Part model, mm, in its own coordinate system. Face numbers are marked on the shaded views. A direction names the side the tool comes from. Round coordinates to 2 decimals unless told otherwise and drop trailing zeros. Loops run counter-clockwise (first coordinate to the right, second up) from the corner with the lowest first, then second, coordinate; pieces in that order, holes last. Notation, with made-up numbers: M 61.25,7 L 81.25,7 A22 ccw 81.25,22 Z; hole C -36,14.25 d2. An arc over 180 degrees is marked long. Answer as CSV lines item,"result". Start each with the question number.
Item 1: Which spindle directions (+Z, -Z, +X, -X, +Y, -Y) get a long thin tool onto all of the face, cutting with end or side? Do the marked faces 4 and 5. Say none if no direction does.
Item 2: Band-saw the part on D-D (z = 5.25). Give the cut face in (x, y).
Item 3: Band-saw the part on C-C (z = 0.5). Give the cut face in (x, y), and give its area (3 significant figures).
Item 4: Band-saw the part on A-A (x = 0). Give the cut face in (y, z), and give its area (3 significant figures).
Item 5: Wall check: line 1 (Y direction, x = 0, z = 2); line 2 (Z direction, x = -4.75, y = -4.25); line 3 (Z direction, x = -4.75, y = 5). Give the ranges that are in metal, low to high.
Item 6: Mould opens along Y. For the marked faces 1, 2 and 3 say: pulls with the +Y half, pulls with the -Y half, needs draft (parallel to the pull), parting line crosses it, or undercut.
Item 7: Drop flat-ended pins along their axis: pin 1 Ø2 at (x, z) = (-4, 1.5) entering from +Y; pin 2 Ø1 at (y, z) = (-4.5, -1.5) entering from -X; pin 3 Ø2 at (x, z) = (2, -3) entering from +Y. Give the stop position or say it passes through.
```python
from build123d import *


with BuildPart() as f1:
    # F0 (on Front) → F1 (revolve)
    with BuildSketch(Plane.XZ):
        Polygon((-1.8, -6), (-1.8, 0), (-4.8, 0), (-4.8, -2.8), (-4.8, -6), align=None)
        Polygon((-4.8, 2.8), (-4.8, 6), (-7, 6), (-7, 5), align=None)
        Polygon((-1.8, 6), (-4.8, 6), (-4.8, 2.8), (-4.8, 0), (-1.8, 0), align=None)
        Polygon((-4.8, -6), (-4.8, -2.8), (-7, -5), (-7, -6), align=None)
    revolve(axis=Axis((0, 0, -0.768788), (0, 0, -1)))


solid = f1.part
```
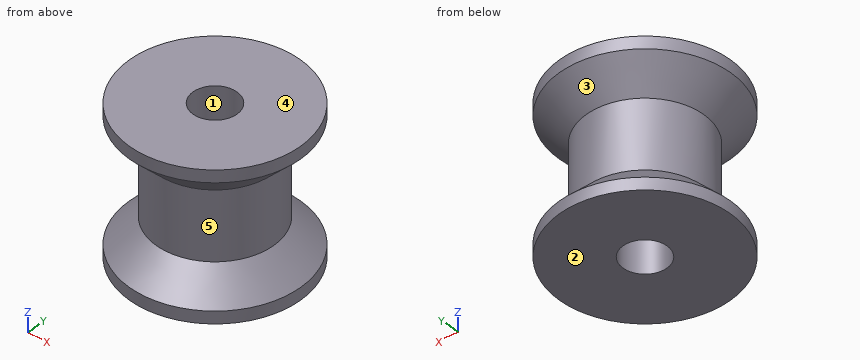
Answer block:
1,face 4,"+Z, +X, -X, +Y, -Y"
1,face 5,"none"
2,outline,"C 0,0 d14; hole C 0,0 d3.6"
3,outline,"C 0,0 d9.6; hole C 0,0 d3.6"
3,area,"62.2 mm^2"
4,outline,"M -7,-6 L -1.8,-6 L -1.8,6 L -7,6 L -7,5 L -4.8,2.8 L -4.8,-2.8 L -7,-5 Z; M 1.8,-6 L 7,-6 L 7,-5 L 4.8,-2.8 L 4.8,2.8 L 7,5 L 7,6 L 1.8,6 Z"
4,area,"90.5 mm^2"
5,line 1,"y = -4.8 to -1.8, 1.8 to 4.8"
5,line 2,"z = -6 to -4.37, 4.37 to 6"
5,line 3,"z = -6 to -4.9, 4.9 to 6"
6,face 1,"undercut"
6,face 2,"needs draft"
6,face 3,"parting line crosses it"
7,pin 1,"stops at y = 3.75"
7,pin 2,"stops at x = -2.65"
7,pin 3,"stops at y = 5.71"
